from build123d import *

# Parameters (mm, degrees)
F1_DEPTH = 609.6
F2_T     = -76.2
F3_DEPTH = 635


with BuildPart() as f1:
    # F0 (on Right) → F1 (new body)
    with BuildSketch(Plane.YZ):
        Polygon((914.4, -457.2), (914.4, 457.2), (-914.4, 457.2), (-914.4, -457.2), (-558.8, -457.2), (-514.805909, -381), (-399.594091, -381), (-355.6, -457.2), (355.6, -457.2), (399.594091, -381), (514.805909, -381), (558.8, -457.2), align=None)
    extrude(amount=F1_DEPTH)

    # F2
    f2_openings = [f1.faces().sort_by_distance(p)[0] for p in [
        (304.8, 0, 457.2),
    ]]
    offset(amount=F2_T, openings=f2_openings)

    # F0 (on Right) → F3 (join)
    with BuildSketch(Plane.YZ):
        Polygon((914.4, -457.2), (914.4, 457.2), (-914.4, 457.2), (-914.4, -457.2), (-558.8, -457.2), (-514.805909, -381), (-399.594091, -381), (-355.6, -457.2), (355.6, -457.2), (399.594091, -381), (514.805909, -381), (558.8, -457.2), align=None)
    extrude(amount=F3_DEPTH)


solid = f1.part
Check sheet for the modelled part. Datum: model origin and axes. Units: mm. A direction names the side the tool comes from. Give positions to 0.01 mm unless a question says otherwise; leave off trailing zeros. Write item = value, one per line.
Item 1: Release check for a two-part mould opening along Y. For faces 1 (the flat face through (313, 734, -457.2)), 2 (the flat face through (313, 914.4, -6)), 3 (the flat face through (313, -914.4, 6)), 4 (the flat face through (313.055, -377.905, -418.567)) record: +Y half, -Y half, draft (parallel to the pull), parting line (faces both ways), or undercut.
Output:
face_1 = draft
face_2 = +Y half
face_3 = -Y half
face_4 = undercut
Item 2: Scan line: probe 1 along Z at (x, y) = (99, 416.5). Record every from-to range of solid material in increasing order. Write a range as from..to.
Output:
probe_1 = -381..457.2
Item 3: Tool access check on faces 5 (the flat face through (313, -458, -381)), 6 (the flat face through (313, 13, 457.2)). Record the directions out of +Z, -Z, +X, -X, +Y, -Y that give a thin tool (end or side, any length) a straight path to the whole face; none if there is none.
Output:
face_5 = -Z, +X, -X
face_6 = +Z, +X, -X, +Y, -Y
